```python
from build123d import *

# Parameters (mm, degrees)
SKETCH1_W           = 14
SKETCH1_H           = 14
BOSS_EXTRUDE1_DEPTH = 4
SKETCH2_W           = 25
SKETCH2_H           = 25
SKETCH2_R           = 1.2446
BOSS_EXTRUDE2_DEPTH = 10
SKETCH3_R           = 4.23
CUT_EXTRUDE1_DEPTH  = 9.8
SKETCH5_R           = 0.6604
CUT_EXTRUDE2_DEPTH  = 14


with BuildPart() as part:
    # Sketch1 → Boss-Extrude1 (new body)
    with BuildSketch(Plane(origin=(0, 0, 0), x_dir=(1, 0, 0), z_dir=(0, 1, 0))):
        Rectangle(SKETCH1_W, SKETCH1_H)
    extrude(amount=BOSS_EXTRUDE1_DEPTH)

    # Sketch2 → Boss-Extrude2 (add)
    with BuildSketch(Plane.XZ):
        Rectangle(SKETCH2_W, SKETCH2_H)
        with Locations((-9.75, 9.75)):
            Circle(SKETCH2_R, mode=Mode.SUBTRACT)
        with Locations((9.75, 9.75)):
            Circle(SKETCH2_R, mode=Mode.SUBTRACT)
        with Locations((9.75, -9.75)):
            Circle(SKETCH2_R, mode=Mode.SUBTRACT)
        with Locations((-9.75, -9.75)):
            Circle(SKETCH2_R, mode=Mode.SUBTRACT)
    extrude(amount=BOSS_EXTRUDE2_DEPTH)

    # Sketch3 → Cut-Extrude1 (cut)
    with BuildSketch(Plane.XZ.offset(10)):
        Circle(SKETCH3_R)
    extrude(amount=-CUT_EXTRUDE1_DEPTH, mode=Mode.SUBTRACT)

    # Sketch4 → Revolve1 (revolve)
    with BuildSketch(Plane(origin=(0, 0, 0), x_dir=(0, 0, -1), z_dir=(1, 0, 0))):
        Polygon((0.6604, 11), (0.6604, 4), (1.6, 4), (1.6, 10.5), (1.1, 11), align=None)
    revolve(axis=Axis((0, 4, 0), (0, 1, 0)))

    # Sketch5 → Cut-Extrude2 (cut)
    with BuildSketch(Plane(origin=(0, 4, 0), x_dir=(1, 0, 0), z_dir=(0, 1, 0))):
        Circle(SKETCH5_R)
    extrude(amount=-CUT_EXTRUDE2_DEPTH, mode=Mode.SUBTRACT)


solid = part.part
```
Check sheet for the modelled part. Datum: model origin and axes. Units: mm. A direction names the side the tool comes from. Round coordinates to 2 decimals unless told otherwise and drop trailing zeros. Write each loop counter-clockwise with the first axis right and the second up, starting at its lowest first coordinate (ties: lowest second). Pieces come first, ordered by that corner, then holes. Notation, with made-up numbers: M 67,-7.75 L 90,-7.75 A28 ccw 90,12.25 Z; hole C 55,86.25 d5. An arc over 180 degrees is marked long. Write item = value, one per line. Start each with the question number.
1. Section check C-C, the plane x = -9.75. Record the cut outline in (y, z), then the cut area to 3 significant figures.
2. Tool access check on faces 5 (the flat face through (7, 2, 0)), 6 (the flat face through (0, 2, -7)), 7 (the cylindrical face through (-10.738, -4.93, 8.993)), 8 (the flat face through (-9, 0, 0)), 9 (the cylindrical face through (-3.36, -5.17, -2.57)). Record the directions out of +Z, -Z, +X, -X, +Y, -Y that give a thin tool (end or side, any length) a straight path to the whole face; none if there is none.
3. Scan lines: line 1 (X direction, y = 1.3, z = 0); line 2 (Y direction, x = -2.5, z = -2.5). Record each from-to range of solid material in increasing order. Write a range as [from, to].
4. Release check for a two-part mould opening along X. For faces 1 (the cylindrical face through (0.97, 7.3, 1.27)), 2 (the flat face through (0, 2, 7)), 3 (the cylindrical face through (-10.738, -4.93, -10.507)), 4 (the flat face through (-7, 2, 0)) record: pulls with the +X half, pulls with the -X half, needs draft (parallel to the pull), parting line crosses it, or undercut.
5. Gauge pin test, flat ends, axial feed: pin 1 (2.5 mm diameter, centred on x = 1, z = 0, fed in from -Y); pin 2 (5 mm diameter, centred on x = -1, y = 8, fed in from +Z); pin 3 (1.5 mm diameter, centred on x = 0, z = 0, fed in from +Y); pin 4 (4 mm diameter, centred on x = 5, z = 7, fed in from +Y). Record the tip position at first contact, or that the pin passes through.
6. Section check B-B, the plane y = -8.5. Record the cut outline in (x, z).
7. Section check D-D, the plane z = -9.75. Record the cut outline in (x, y), then the cut area to 3 significant figures.
8. Section check A-A, the plane z = 0. Record the cut outline in (x, y), then the cut area to 3 significant figures.
Results found:
q1.outline = M -10,-12.5 L 0,-12.5 L 0,-10.99 L -10,-10.99 Z; M -10,-8.51 L 0,-8.51 L 0,8.51 L -10,8.51 Z; M -10,10.99 L 0,10.99 L 0,12.5 L -10,12.5 Z
q1.area = 200 mm^2
q2.face_5 = +Z, -Z, +X, +Y
q2.face_6 = -Z, +X, -X, +Y
q2.face_7 = +Y, -Y
q2.face_8 = +Y
q2.face_9 = -Y
q3.line_1 = [-7, -0.66], [0.66, 7]
q3.line_2 = [-0.2, 4]
q4.face_1 = parting line crosses it
q4.face_2 = needs draft
q4.face_3 = undercut
q4.face_4 = pulls with the -X half
q5.pin_1 = -0.2
q5.pin_2 = 1.6
q5.pin_3 = 11
q5.pin_4 = 4
q6.outline = M -12.5,-12.5 L 12.5,-12.5 L 12.5,12.5 L -12.5,12.5 Z; hole C -9.75,-9.75 d2.49; hole C -9.75,9.75 d2.49; hole C 0,0 d8.46; hole C 9.75,-9.75 d2.49; hole C 9.75,9.75 d2.49
q7.outline = M -12.5,-10 L -10.99,-10 L -10.99,0 L -12.5,0 Z; M -8.51,-10 L 8.51,-10 L 8.51,0 L -8.51,0 Z; M 10.99,-10 L 12.5,-10 L 12.5,0 L 10.99,0 Z
q7.area = 200 mm^2
q8.outline = M -12.5,-10 L -4.23,-10 L -4.23,-0.2 L -0.66,-0.2 L -0.66,11 L -1.1,11 L -1.6,10.5 L -1.6,4 L -7,4 L -7,0 L -12.5,0 Z; M 0.66,-0.2 L 4.23,-0.2 L 4.23,-10 L 12.5,-10 L 12.5,0 L 7,0 L 7,4 L 1.6,4 L 1.6,10.5 L 1.1,11 L 0.66,11 Z
q8.area = 230 mm^2
